CAD build for the part. Positions are in the model's coordinates, mm. A direction names the side the tool comes from. Coordinates: 2 decimals unless noted, no trailing zeros. Order: outer loops, then holes, each group sorted by start corner. A loop starts at its lowest first (then second) coordinate and runs counter-clockwise, first axis right, second up. Notation, with made-up numbers: (18, 0.5) - (50, 0.5) arc R28 ccw to (50, 27.5) - close; hole circle Ø8 at (75.5, -16.5). An arc over 180 degrees is marked (long way). Write each question's results on one line, items separated by ' | '. Start each with the question number.
Q1. Band-saw the part on C-C, the plane x = 15. Write the cut outline in (y, z) (3 decimals).
Q2. Band-saw the part on B-B, the plane y = 0. Write the cut outline in (x, z).
Q3. Band-saw the part on D-D, the plane z = 3.5. Write the cut outline in (x, y) (3 decimals).
Q4. Wall check: probe 1 along Y at (x, z) = (15, 2.25) (3 decimals); probe 2 along Y at (x, z) = (0, 1.6); probe 3 along Z at (x, y) = (-2, 8.25). Give the ranges that are in metal, low to high.
Q5. Pin check, flat tips, straight feed: P1, Ø12, axis at x = 7, y = -2.5, coming from the +Z side; P2, Ø5, axis at y = 8.5, z = 10, coming from the +X side; P3, Ø2.5, axis at x = 15, y = 10, coming from the -Z side. Stop position of each tip, or through.
Q6. Pull direction X, two halves, no side cores. Call faces 4 (the cylindrical face through (13.31, 11.29, 2.46)), 5 (the flat face through (20, 0, 2)), 6 (the flat face through (-4, 15, 4)), 7 (the cylindrical face through (-1.08, 4.88, 2.46)): released by +X, released by -X, zero draft, split by the parting line, or undercut.
Q7. Band-saw the part on A-A, the plane x = 0. Write the cut outline in (y, z).
Q8. Which spindle directions (+Z, -Z, +X, -X, +Y, -Y) get a long thin tool onto all of the face, cutting with end or side? Do faces 1 (the flat face through (-14, 2.5, 10)), 2 (the cylindrical face through (13.31, -8.71, 2.46)), 3 (the flat face through (-7.5, 9, 10)). Say none if no direction does.
Autodesk Inventor part; units mm, degrees
ref_plane "YZ Plane" through (0, 0, 0) normal (1, 0, 0) x (0, 1, 0)
ref_plane "XZ Plane" through (0, 0, 0) normal (0, 1, 0) x (-1, 0, 0)
ref_plane "XY Plane" through (0, 0, 0) normal (0, 0, 1) x (1, 0, 0)
sketch "Sketch1" plane through (0, 0, 0) normal (0, 0, 1) x (1, 0, 0)
  line L0 (20, 15) -> (-20, 15)
  line L1 (-20, 15) -> (-20, -15)
  line L2 (-20, -15) -> (20, -15)
  line L3 (20, -15) -> (20, 15)
  line L4 (0, 0) -> (1.9807, 0) construction
  line L5 (0, 0) -> (0, -2.0582) construction
  circle A0 centre (15, -10) radius 2.125
  circle A1 centre (15, 10) radius 2.125
  circle A2 centre (0, 0) radius 2.125
  circle A3 centre (15, -10) radius 2.125
  circle A4 centre (15, 10) radius 2.125
  circle A5 centre (0, 0) radius 2.125
  circle A6 centre (0, 0) radius 2.125
  circle A7 centre (0, 0) radius 5
  dimension "d4" = 40
  dimension "d5" = 30
  dimension "d8" = 10
extrude "Extrusion1" add sketch "Sketch1" along normal blind 5 contours L3 L2 L1 L0
sketch "Sketch3" plane through (0, 0, 5) normal (0, 0, 1) x (1, 0, 0)
  line L0 (-20, -15) -> (20, -15)
  line L1 (20, -15) -> (20, 15)
  line L2 (20, 15) -> (-20, 15)
  line L3 (-7.5, -15) -> (-7.5, -2.5)
  line L4 (-7.5, -2.5) -> (-20, -2.5)
  line L5 (-20, 15) -> (-20, -15)
  line L6 (-20, 2.5) -> (-7.5, 2.5)
  line L7 (-7.5, 2.5) -> (-7.5, 15)
  point P0 (0, 0)
  dimension "d9" = 5
extrude "Extrusion2" add sketch "Sketch3" along normal blind 10 contours L5 L4 L3 L0 | L5 L2 L7 L6
properties part number "YCartBeltClamp"
Results below:
1) outline: (-15, 0) - (-12.125, 0) - (-12.125, 5) - (-15, 5) - close; (-7.875, 0) - (7.875, 0) - (7.875, 5) - (-7.875, 5) - close; (12.125, 0) - (15, 0) - (15, 5) - (12.125, 5) - close
2) outline: (-20, 0) - (-5, 0) - (-5, 5) - (-20, 5) - close; (5, 0) - (20, 0) - (20, 5) - (5, 5) - close
3) outline: (-20, -15) - (20, -15) - (20, 15) - (-20, 15) - close; hole circle Ø10 at (0, 0); hole circle Ø4.25 at (15, -10); hole circle Ø4.25 at (15, 10)
4) probe 1: y = -15 to -12.125, -7.875 to 7.875, 12.125 to 15 | probe 2: y = -15 to -5, 5 to 15 | probe 3: z = 0 to 5
5) P1: stops at z = 5 | P2: stops at x = -7.5 | P3: passes through
6) face 4: undercut | face 5: released by +X | face 6: zero draft | face 7: undercut
7) outline: (-15, 0) - (-5, 0) - (-5, 5) - (-15, 5) - close; (5, 0) - (15, 0) - (15, 5) - (5, 5) - close
8) face 1: +Z, +X, -X | face 2: +Z, -Z | face 3: +Z, +X, +Y, -Y
